The figure shows three views and two pictorial views of one solid part (mm, origin at its lowest corner). Answer the questions. A direction names the side the tool comes from. Give positions to 0.01 mm unless a question says otherwise; leave off trailing zeros. Loops run counter-clockwise (first coordinate to the right, second up) from the corner with the lowest first, then second, coordinate; pieces in that order, holes last. Notation, with made-up numbers: M 55,-23 L 85,-23 A10 cw 85,-11 Z; hole C 84,-16 d1. An arc over 180 degrees is marked long. Answer in a Markdown table with one row per item. Add a question column.
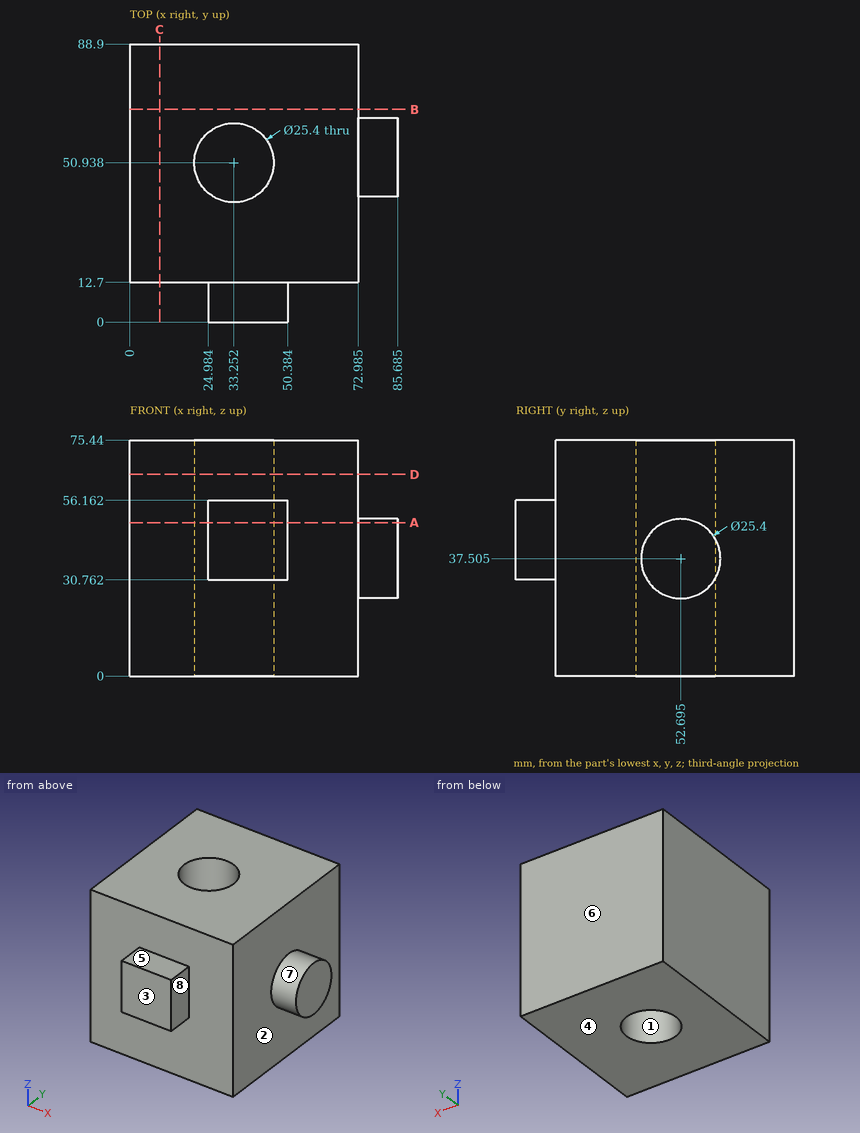
(1) Section C-C, the plane x = 9.5 is taken. Determine the outline of the cut face in (y, z).
(2) The mould has two halves that part along Y. Classify the marked faces 1, 2 and 3: pulls with the +Y half, pulls with the -Y half, needs draft (parallel to the pull), parting line crosses it, or undercut.
(3) Each of these flat-tipped pins is pushed along its axis until it touches: P1, Ø6.5, axis at y = 6, z = 44, coming from the -X side; P2, Ø6.5, axis at y = 9, z = 46, coming from the +X side; P3, Ø10, axis at y = 32.5, z = 61.5, coming from the +X side (1 decimal). Where does it stop, or does it pass through?
(4) Which of the six approach directions +Z, -Z, +X, -X, +Y, -Y give full straight-line access (tool end or side, diameter ignored) to the marked faces 4, 5, 6, 7 and 8?
(5) Section A-A, the plane z = 49 is taken. Determine the outline of the cut face in (x, y) (1 decimal), and give its area (3 significant figures).
(6) Consider line 1 along Y through (x, z) = (47.5, 29.5); line 2 along X through (y, z) = (34, 46) (1 decimal); line 3 along Y through (x, z) = (38.5, 8). Determine where each line is inside the solid, lowest interval first. Write a range as from..to.
(7) Section B-B, the plane y = 68 is taken. Determine the outline of the cut face in (x, z) (1 decimal).
(8) Section D-D, the plane z = 64.5 is taken. Determine the outline of the cut face in (x, y) (1 decimal).
Numbers:
| question | item | result |
|---|---|---|
| 1 | outline | M 12.7,0 L 88.9,0 L 88.9,75.44 L 12.7,75.44 Z |
| 2 | face 1 | undercut |
| 2 | face 2 | needs draft |
| 2 | face 3 | pulls with the -Y half |
| 3 | P1 | stops at x = 24.98 |
| 3 | P2 | stops at x = 50.38 |
| 3 | P3 | stops at x = 73 |
| 4 | face 4 | -Z, +X, -X, +Y, -Y |
| 4 | face 5 | +Z, +X, -X, -Y |
| 4 | face 6 | +Z, -Z, +X, -X, +Y |
| 4 | face 7 | +X |
| 4 | face 8 | +Z, -Z, +X, -Y |
| 5 | outline | M 0,12.7 L 25,12.7 L 25,0 L 50.4,0 L 50.4,12.7 L 73,12.7 L 73,47.3 L 85.7,47.3 L 85.7,58.1 L 73,58.1 L 73,88.9 L 0,88.9 Z; hole C 33.3,50.9 d25.4 |
| 5 | area | 5,510 mm² |
| 6 | line 1 | y = 12.7..88.9 |
| 6 | line 2 | x = 0..73 |
| 6 | line 3 | y = 12.7..39.37, 62.5..88.9 |
| 7 | outline | M 0,0 L 73,0 L 73,75.4 L 0,75.4 Z |
| 8 | outline | M 0,12.7 L 73,12.7 L 73,88.9 L 0,88.9 Z; hole C 33.3,50.9 d25.4 |
